Here's the drawing with two shaded views (mm, measured from the low corner). I have some questions. Round coordinates to 2 decimals unless told otherwise and drop trailing zeros. Loops run counter-clockwise (first coordinate to the right, second up) from the corner with the lowest first, then second, coordinate; pieces in that order, holes last. Notation, with made-up numbers: M -35,24.25 L 3,24.25 A19 cw 3,45.25 Z; hole C -26,-8.5 d8. An arc over 180 degrees is marked long. One line per item, written item: value. Start each with the question number.
Q1. Imagine slicing it at A-A (z = 0.95). Please give me the cut outline in (x, y), then the cut area to 3 significant figures.
Q2. Imagine slicing it at C-C (x = 20). Please give me the cut outline in (y, z), then the cut area to 3 significant figures.
Q3. I'm going to push flat-ended pins straight in: pin 1 Ø1.5 at (x, z) = (31.5, 2) entering from -Y; pin 2 Ø2.5 at (x, y) = (5, 9) entering from -Z. Where does each tip first touch, or does it pass through?
Q4. Please list where these lines run through material, in increasing order: line 1 along Y through (x, z) = (20, 1.95); line 2 along Y through (x, z) = (28.5, 2.85); line 3 along X through (y, z) = (33.5, 2.4).
Q5. Thinking about a two-plate mould opening in X: for the marked faces 1, 2 and 3, which applies, released by +X, released by -X, zero draft, split by the parting line, or undercut?
Q6. Imagine slicing it at B-B (y = 9). Please give me the cut outline in (x, z), then the cut area to 3 significant figures.
Q7. Imagine slicing it at D-D (x = 24). Please give me the cut outline in (y, z), then the cut area to 3 significant figures.
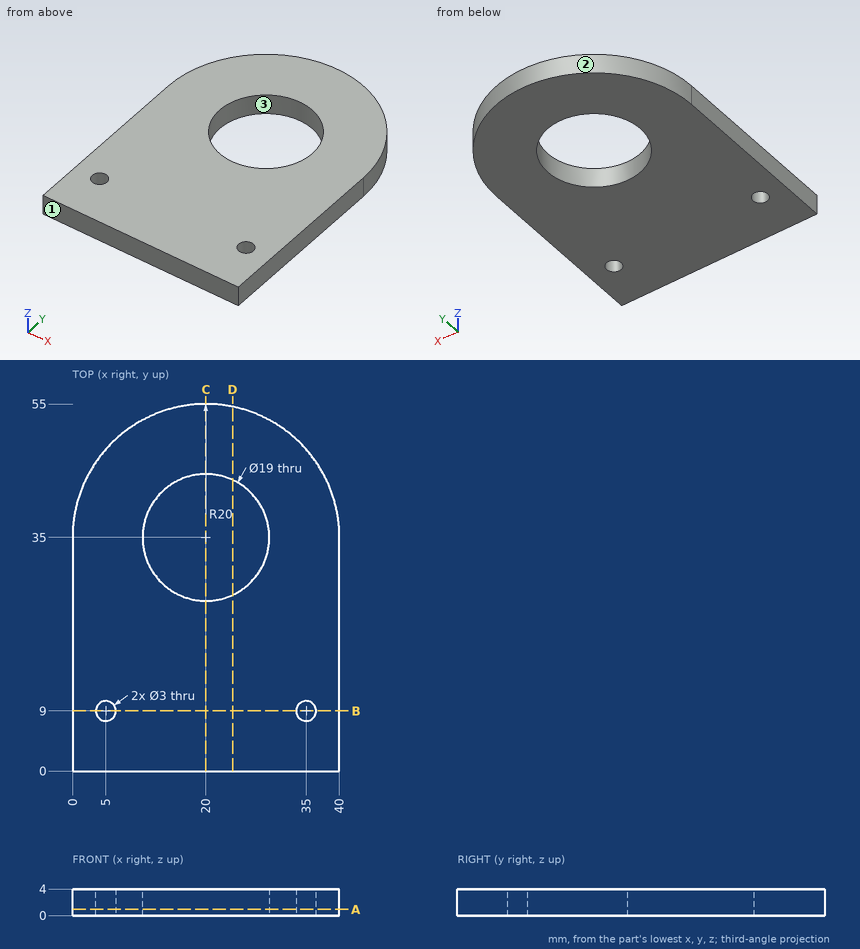
Report:
1. outline: M 0,0 L 40,0 L 40,35 A20 ccw 0,35 Z; hole C 5,9 d3; hole C 20,35 d19; hole C 35,9 d3
1. area: 1,730 mm²
2. outline: M 0,0 L 25.5,0 L 25.5,4 L 0,4 Z; M 44.5,0 L 55,0 L 55,4 L 44.5,4 Z
2. area: 144 mm²
3. pin 1: stops at y = 0
3. pin 2: passes through
4. line 1: y = 0 to 25.5, 44.5 to 55
4. line 2: y = 0 to 30.76, 39.24 to 53.1
4. line 3: x = 0 to 10.62, 29.38 to 40
5. face 1: zero draft
5. face 2: split by the parting line
5. face 3: undercut
6. outline: M 0,0 L 3.5,0 L 3.5,4 L 0,4 Z; M 6.5,0 L 33.5,0 L 33.5,4 L 6.5,4 Z; M 36.5,0 L 40,0 L 40,4 L 36.5,4 Z
6. area: 136 mm²
7. outline: M 0,0 L 26.38,0 L 26.38,4 L 0,4 Z; M 43.62,0 L 54.6,0 L 54.6,4 L 43.62,4 Z
7. area: 149 mm²
